For this review, take the finished solid that the model builds, in its own axes (mm). Face numbers are marked on the shaded views. A direction names the side the tool comes from. Coordinates: 2 decimals unless noted, no trailing zeros. Loops run counter-clockwise (first coordinate to the right, second up) from the corner with the lowest first, then second, coordinate; pieces in that order, holes last. Notation, with made-up numbers: M 79.5,-33.75 L 128.5,-33.75 A15 ccw 128.5,-23.75 Z; hole C -29,28 d3. An arc over 180 degrees is marked long. Write each question's results on one line, items separated by ' | '. Start each with the question number.
```python
from build123d import *

# Parameters (mm, degrees)
F0_W     = 609.6
F0_H     = 609.6
F1_DEPTH = 50.8
F4_R     = 25.4
F5_DEPTH = 50.801


with BuildPart() as f1:
    # F0 (on Top) → F1 (new body)
    with BuildSketch(Plane.XY):
        Rectangle(F0_W, F0_H)
    extrude(amount=F1_DEPTH)

    # F2 (on Front) → F3 (revolve)
    with BuildSketch(Plane.XZ):
        Polygon((152.4, 101.6), (101.6, 50.8), (203.2, 50.8), (203.2, 101.6), align=None)
    revolve(axis=Axis((0, 0, 25.4), (0, 0, 1)))

    # F4 (on face) → F5 (cut, through all)
    with BuildSketch(Plane.XY.offset(50.8)):
        with Locations((-228.6, 228.6)):
            Circle(F4_R)
        with Locations((228.6, 228.6)):
            Circle(F4_R)
        with Locations((228.6, -228.6)):
            Circle(F4_R)
        with Locations((-228.6, -228.6)):
            Circle(F4_R)
    extrude(amount=-F5_DEPTH, mode=Mode.SUBTRACT)


solid = f1.part
```
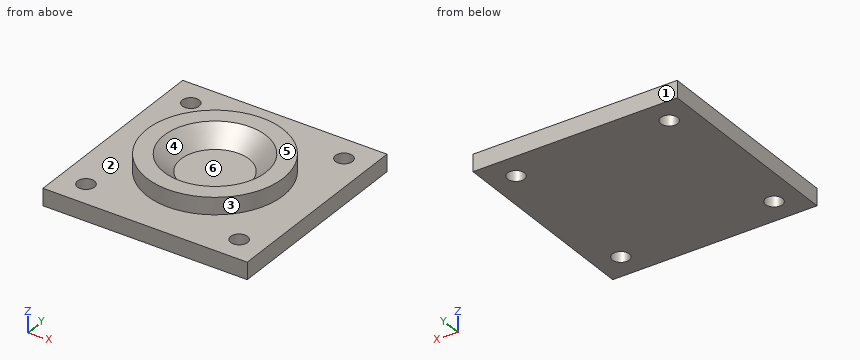
Q1. Take a section at D-D, the plane z = 41. Give the boundary of the cut face in (x, y), then the cut area to 3 significant figures.
Q2. The part is to be moulded in two halves that separate along X. For the marked faces 3, 4, 5 and 6, say which applies: pulls with the +X half, pulls with the -X half, needs draft (parallel to the pull), parting line crosses it, or undercut.
Q3. Take a section at A-A, the plane x = -228.6. Give the boundary of the cut face in (y, z), then the cut area to 3 significant figures.
Q4. To check wall thickness, follow line 1 along Y through (x, z) = (228, 31); line 2 along Z through (x, y) = (206, -104). State the ranges of each line that lie inside material, in increasing order.
Q5. Insertion check: P1, Ø10, axis at x = 52, y = 134, coming from the -Z side; P2, Ø4, axis at x = 138.5, z = 57.5, coming from the -Y side; P3, Ø5, axis at x = -44, z = 58.5, coming from the +Y side; P4, Ø6, axis at x = -149, z = 66.5, coming from the +Y side. Each pin has a flat end and moves straight along its axis. Give the tip position at first contact, or say it passes through.
Q6. For the marked faces 1 and 2, list the 3-axis set-ups (+Z, -Z, +X, -X, +Y, -Y) from which the entire face can be reached by the end or side of a thin tool; tool diameter is ignored.
Q7. Take a section at C-C, the plane x = 0. Give the boundary of the cut face in (y, z).
Results:
1) outline: M -304.8,-304.8 L 304.8,-304.8 L 304.8,304.8 L -304.8,304.8 Z; hole C -228.6,-228.6 d50.8; hole C -228.6,228.6 d50.8; hole C 228.6,-228.6 d50.8; hole C 228.6,228.6 d50.8 | area: 364,000 mm^2
2) face 3: parting line crosses it | face 4: undercut | face 5: needs draft | face 6: undercut
3) outline: M -304.8,0 L -254,0 L -254,50.8 L -304.8,50.8 Z; M -203.2,0 L 203.2,0 L 203.2,50.8 L -203.2,50.8 Z; M 254,0 L 304.8,0 L 304.8,50.8 L 254,50.8 Z | area: 25,800 mm^2
4) line 1: -304.8 to -253.99, -203.21 to 203.21, 253.99 to 304.8 | line 2: 0 to 50.8
5) P1: z = 0 | P2: y = -150.53 | P3: y = 198.92 | P4: y = 141.33
6) face 1: +Z, -Z, +X, -X, +Y | face 2: +Z
7) outline: M -304.8,0 L 304.8,0 L 304.8,50.8 L 203.2,50.8 L 203.2,101.6 L 152.4,101.6 L 101.6,50.8 L -101.6,50.8 L -152.4,101.6 L -203.2,101.6 L -203.2,50.8 L -304.8,50.8 Z
